Can you work these out from the model? Positions are in its coordinate system, mm. Face numbers are marked on the shaded views. A direction names the side the tool comes from. Round coordinates to 2 decimals unless told otherwise and drop trailing zeros. Write each loop counter-clockwise with the first axis right and the second up, starting at its lowest first coordinate (ties: lowest second). Pieces come first, ordered by that corner, then holes. Notation, with made-up numbers: (17, 6) -> (36, 6) arc R28 ccw to (36, 32) -> close; hole circle Ø4 at (-31.75, -39). An arc over 180 degrees is marked (long way). Write item = value, one per line. Start each with the question number.
1) Imagine slicing it at B-B, the plane x = 28. Please give me the cut outline in (y, z), then the cut area to 3 significant figures.
2) If I drill on line 1 (Z direction, x = 31, y = 43); line 2 (Z direction, x = -25.5, y = 48); line 3 (Y direction, x = 0, z = -13), over which ranges is the centre line in solid material (lowest first)?
3) Imagine slicing it at D-D, the plane x = 0. State how many separate pieces and enclosed holes the cut face has, then the cut area to 3 significant figures.
4) Imagine slicing it at A-A, the plane z = 7. Please give me the cut outline in (x, y).
5) Thinking about a two-plate mould opening in X: for the marked faces 1, 2 and 3, which applies, +X half, -X half, draft (parallel to the pull), parting line (faces both ways), or undercut?
6) For the marked faces 4, 5 and 6, which set-ups out of +Z, -Z, +X, -X, +Y, -Y let a thin tool reach every point of the face, with its end or its side?
7) Imagine slicing it at C-C, the plane z = -7. Please give me the cut outline in (x, y).
8) I'm going to push flat-ended pins straight in: pin 1 (8 mm diameter, centred on x = 10.5, y = 55.5, fed in from +Z); pin 2 (7.5 mm diameter, centred on x = -1, y = 82.5, fed in from +Z); pin 3 (3 mm diameter, centred on x = 8, z = -8, fed in from +Y). Where does each tip first touch, or does it pass through?
from build123d import *

# Parameters (mm, degrees)
BOSS_EXTRUDE2_DEPTH = 87
SHELL2_T            = -3
SKETCH3_W           = 3
SKETCH3_H           = 3
BOSS_EXTRUDE3_DEPTH = 84
CUT_EXTRUDE1_REACH  = 106.538
SKETCH4_R           = 3.3
CUT_EXTRUDE2_REACH  = 107.796
SKETCH5_R           = 6.3
SKETCH5_R_2         = 2.8
BOSS_EXTRUDE4_DEPTH = 84
CUT_EXTRUDE3_REACH  = 102.465
SKETCH7_W           = 7.5
SKETCH7_H           = 3.7
SKETCH8_R           = 3.7
BOSS_EXTRUDE5_DEPTH = 8
SKETCH9_R           = 1.8
CUT_EXTRUDE4_DEPTH  = 11
SKETCH10_R          = 5.3
CUT_EXTRUDE5_DEPTH  = 1.8
SKETCH11_R          = 5.3
CUT_EXTRUDE6_DEPTH  = 1.8
CUT_EXTRUDE7_REACH  = 101.657
SKETCH15_R          = 3.5
CUT_EXTRUDE8_START  = -1.5
SKETCH17_R          = 3.5
CUT_EXTRUDE8_DEPTH  = 1.5
SKETCH18_W          = 68.6
SKETCH18_H          = 3
CUT_EXTRUDE9_DEPTH  = 1
SKETCH31_W          = 3
SKETCH31_H          = 8.317693095
BOSS_EXTRUDE6_DEPTH = 8
CUT_EXTRUDE10_DEPTH = 3


with BuildPart() as part:
    # Sketch1 → Boss-Extrude2 (new body)
    with BuildSketch(Plane(origin=(0, 0, 0), x_dir=(1, 0, 0), z_dir=(0, 1, 0))):
        Polygon((-29.3, 14.3), (-29.3, -31.3), (-14.3, -31.3), (2.7, -14.3), (34.3, -14.3), (34.3, -31.3), (39.3, -31.3), (39.3, -2.7), (29.3, -2.7), (29.3, 2.7), (39.3, 2.7), (39.3, 14.3), align=None)
    extrude(amount=BOSS_EXTRUDE2_DEPTH)

    # Shell2
    shell2_openings = [part.faces().sort_by_distance(p)[0] for p in [
        (1.788570481, 87, 4.446127974),
    ]]
    offset(amount=SHELL2_T, openings=shell2_openings, kind=Kind.INTERSECTION)

    # Sketch3 → Boss-Extrude3 (add)
    with BuildSketch(Plane(origin=(0, 3, 0), x_dir=(1, 0, 0), z_dir=(0, 1, 0))):
        with Locations((24.8, 2.8)):
            Rectangle(SKETCH3_W, SKETCH3_H)
        with Locations((24.8, -2.8)):
            Rectangle(SKETCH3_W, SKETCH3_H)
        with Locations((-24.8, -2.8)):
            Rectangle(SKETCH3_W, SKETCH3_H)
        with Locations((-24.8, 2.8)):
            Rectangle(SKETCH3_W, SKETCH3_H)
    extrude(amount=BOSS_EXTRUDE3_DEPTH)

    # Cut-Extrude1: up to this face of the body (flat: up to its plane)
    cut_extrude1_end = Plane(part.part.faces().sort_by_distance((31.3, 45, 5.7))[0])
    # Sketch4 → Cut-Extrude1 (cut, up to the picked face)
    with BuildSketch(Plane.XY.offset(-11.3), mode=Mode.PRIVATE) as cut_extrude1_sk1:
        with Locations(Location((32.8, 77, 0), (0, 0, 180))):
            Circle(SKETCH4_R)
    cut_extrude1_tool1 = split(extrude(cut_extrude1_sk1.sketch, amount=CUT_EXTRUDE1_REACH, mode=Mode.PRIVATE), bisect_by=cut_extrude1_end, keep=Keep.BOTH, mode=Mode.PRIVATE)
    add(cut_extrude1_tool1.solids().sort_by(Axis((32.8, 77, -11.3), (0, 0, 1)))[0], mode=Mode.SUBTRACT)

    # Sketch5 → Cut-Extrude2 (cut, up to next)
    with BuildSketch(Plane(origin=(0, 0, -14.3), x_dir=(-1, 0, 0), z_dir=(0, 0, -1)), mode=Mode.PRIVATE) as cut_extrude2_sk1:
        with Locations((0, 55)):
            Circle(SKETCH5_R)
    cut_extrude2_tool1 = extrude(cut_extrude2_sk1.sketch, amount=-CUT_EXTRUDE2_REACH, mode=Mode.PRIVATE) & part.part
    # Sketch5 → Cut-Extrude2 (cut, up to next)
    with BuildSketch(Plane(origin=(0, 0, -14.3), x_dir=(-1, 0, 0), z_dir=(0, 0, -1)), mode=Mode.PRIVATE) as cut_extrude2_sk2:
        with Locations((0, 71)):
            Circle(SKETCH5_R_2)
    cut_extrude2_tool2 = extrude(cut_extrude2_sk2.sketch, amount=-CUT_EXTRUDE2_REACH, mode=Mode.PRIVATE) & part.part
    add(cut_extrude2_tool1.solids().sort_by_distance((0, 55, -14.3))[0], mode=Mode.SUBTRACT)
    add(cut_extrude2_tool2.solids().sort_by_distance((0, 71, -14.3))[0], mode=Mode.SUBTRACT)

    # Sketch6 → Boss-Extrude4 (add)
    with BuildSketch(Plane(origin=(0, 3, 0), x_dir=(1, 0, 0), z_dir=(0, 1, 0))):
        Polygon((1.457359313, -11.3), (-26.3, -11.3), (-26.3, -28.3), (-15.542640687, -28.3), align=None)
    extrude(amount=BOSS_EXTRUDE4_DEPTH)

    # Sketch7 → Cut-Extrude3 (cut, up to next)
    with BuildSketch(Plane.XZ, mode=Mode.PRIVATE) as cut_extrude3_sk1:
        with Locations((0, -7.15)):
            Rectangle(SKETCH7_W, SKETCH7_H)
    cut_extrude3_tool1 = extrude(cut_extrude3_sk1.sketch, amount=-CUT_EXTRUDE3_REACH, mode=Mode.PRIVATE) & part.part
    add(cut_extrude3_tool1.solids().sort_by_distance((0, 0, -7.15))[0], mode=Mode.SUBTRACT)

    # Sketch8 → Boss-Extrude5 (add)
    with BuildSketch(Plane(origin=(0, 0, 11.3), x_dir=(-1, 0, 0), z_dir=(0, 0, -1))):
        with Locations((0, 81)):
            Circle(SKETCH8_R)
    extrude(amount=BOSS_EXTRUDE5_DEPTH)

    # Sketch9 → Cut-Extrude4 (cut)
    with BuildSketch(Plane(origin=(0, 0, 3.3), x_dir=(-1, 0, 0), z_dir=(0, 0, -1))):
        with Locations((0, 81)):
            Circle(SKETCH9_R)
    extrude(amount=-CUT_EXTRUDE4_DEPTH, mode=Mode.SUBTRACT)

    # Sketch10 → Cut-Extrude5 (cut)
    with BuildSketch(Plane(origin=(8.5, 0, 8.5), x_dir=(0.7071067811865475, 0, -0.7071067811865476), z_dir=(0.7071067811865476, 0, 0.7071067811865475))):
        with Locations((-20.223253942, 43.5)):
            Circle(SKETCH10_R)
    extrude(amount=-CUT_EXTRUDE5_DEPTH, mode=Mode.SUBTRACT)

    # Sketch11 → Cut-Extrude6 (cut)
    with BuildSketch(Plane.ZY.offset(-34.3)):
        with Locations((22.8, 43.5)):
            Circle(SKETCH11_R)
    extrude(amount=-CUT_EXTRUDE6_DEPTH, mode=Mode.SUBTRACT)

    # Cut-Extrude7: up to this face of the body (flat: up to its plane)
    cut_extrude7_end = Plane(part.part.faces().sort_by_distance((-13.661760233, 43.5, 30.661760233))[0])
    # Sketch15 → Cut-Extrude7 (cut, up to the picked face)
    with BuildSketch(Plane(origin=(0, 0, 14.3), x_dir=(-1, 0, 0), z_dir=(0, 0, -1)), mode=Mode.PRIVATE) as cut_extrude7_sk1:
        with Locations((0, 81)):
            Circle(SKETCH15_R)
    cut_extrude7_tool1 = split(extrude(cut_extrude7_sk1.sketch, amount=-CUT_EXTRUDE7_REACH, mode=Mode.PRIVATE), bisect_by=cut_extrude7_end, keep=Keep.BOTH, mode=Mode.PRIVATE)
    add(cut_extrude7_tool1.solids().sort_by(Axis((0, 81, 14.3), (0, 0, 1)))[0], mode=Mode.SUBTRACT)

    # Sketch17 → Cut-Extrude8 (cut)
    with BuildSketch(Plane.XY.offset(14.3).offset(CUT_EXTRUDE8_START)):
        with Locations(Location((0, 81, 0), (0, 0, 39.517652797))):
            Circle(SKETCH17_R)
    extrude(amount=CUT_EXTRUDE8_DEPTH, mode=Mode.SUBTRACT)

    # Sketch18 → Cut-Extrude9 (cut)
    with BuildSketch(Plane(origin=(0, 0, -14.3), x_dir=(-1, 0, 0), z_dir=(0, 0, -1))):
        with Locations((-5, 77)):
            Rectangle(SKETCH18_W, SKETCH18_H)
    extrude(amount=-CUT_EXTRUDE9_DEPTH, mode=Mode.SUBTRACT)

    # Sketch31 → Boss-Extrude6 (add)
    with BuildSketch(Plane(origin=(0, 0, 11.3), x_dir=(-1, 0, 0), z_dir=(0, 0, -1))):
        with Locations((0, 73.458846548)):
            Rectangle(SKETCH31_W, SKETCH31_H)
    extrude(amount=BOSS_EXTRUDE6_DEPTH)

    # Sketch32 → Cut-Extrude10 (cut)
    with BuildSketch(Plane(origin=(1.5, 0, 0), x_dir=(0, 0, -1), z_dir=(1, 0, 0))):
        Polygon((-11.3, 69.3), (-3.3, 77.617693095), (-3.3, 69.3), align=None)
    extrude(amount=-CUT_EXTRUDE10_DEPTH, mode=Mode.SUBTRACT)


solid = part.part
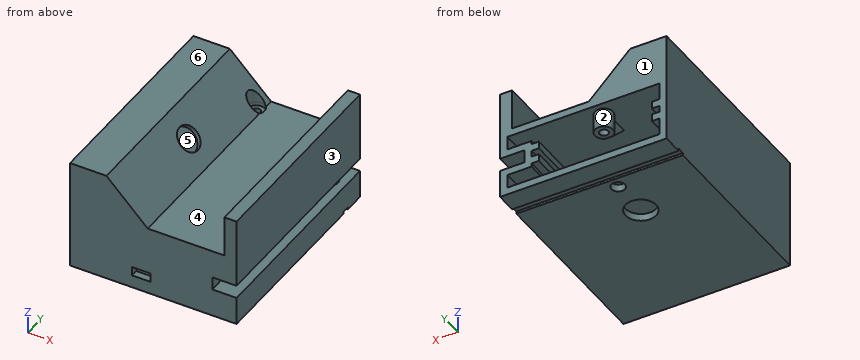
Reported:
q1.outline = (0, -14.3) -> (75.5, -14.3) -> (75.5, -13.3) -> (78.5, -13.3) -> (78.5, -14.3) -> (87, -14.3) -> (87, -11.3) -> (3, -11.3) -> (3, -5.7) -> (87, -5.7) -> (87, 5.7) -> (3, 5.7) -> (3, 11.3) -> (87, 11.3) -> (87, 14.3) -> (0, 14.3) -> close
q1.area = 1,540 mm²
q2.line_1 = -14.3 to -11.3, -5.7 to -2.7, 2.7 to 5.7, 11.3 to 14.3
q2.line_2 = -14.3 to -11.3, -4.3 to -1.3, 1.3 to 4.3, 11.3 to 31.3
q2.line_3 = 0 to 48.7, 61.3 to 68.2, 73.8 to 87
q3.separate_pieces = 5
q3.enclosed_holes = 0
q3.area = 782 mm²
q4.outline = (-29.3, 0) -> (39.3, 0) -> (39.3, 87) -> (36.3, 87) -> (36.3, 3) -> (-26.3, 3) -> (-26.3, 87) -> (-29.3, 87) -> close; (-1.5, 73.77) -> (1.5, 73.77) -> (1.5, 77.62) arc R3.7 ccw (long way) to (-1.5, 77.62) -> close; hole circle Ø3.6 at (0, 81)
q5.face_1 = draft
q5.face_2 = undercut
q5.face_3 = +X half
q6.face_4 = +Z, +Y, -Y
q6.face_5 = none
q6.face_6 = +Z, +X, -X, +Y, -Y
q7.outline = (-29.3, 0) -> (-3.75, 0) -> (-3.75, 3) -> (-26.3, 3) -> (-26.3, 87) -> (-29.3, 87) -> close; (3.75, 0) -> (39.3, 0) -> (39.3, 87) -> (36.3, 87) -> (36.3, 3) -> (3.75, 3) -> close
q8.pin_1 = 14.3
q8.pin_2 = 21.75
q8.pin_3 = 3
